Geometry: final body of the model. Coordinates: model frame, mm. A direction names the side the tool comes from. Give positions to 0.01 mm unless a question says otherwise; leave off trailing zeros. Write each loop counter-clockwise with the first axis right and the second up, starting at its lowest first coordinate (ties: lowest second). Pieces come first, ordered by that corner, then holes.
```python
from build123d import *

# Parameters (mm, degrees)
SKETCH1_W                 = 20
SKETCH1_H                 = 10
BOSS_EXTRUDE1_DEPTH       = 90
M4X0_7_TAPPED_HOLE1_D     = 3.3
M4X0_7_TAPPED_HOLE1_DEPTH = 15
M4X0_7_TAPPED_HOLE1_TIP   = 0.991420021
M4X0_7_TAPPED_HOLE2_D     = 3.3
M4X0_7_TAPPED_HOLE2_DEPTH = 15
M4X0_7_TAPPED_HOLE2_TIP   = 0.991420021


with BuildPart() as part:
    # Sketch1 → Boss-Extrude1 (new body)
    with BuildSketch(Plane(origin=(0, 0, 0), x_dir=(1, 0, 0), z_dir=(0, 1, 0))):
        Rectangle(SKETCH1_W, SKETCH1_H)
    extrude(amount=BOSS_EXTRUDE1_DEPTH)

    # M4x0.7 Tapped Hole1
    with Locations(Plane(origin=(0, 0, 0), x_dir=(-1, 0, 0), z_dir=(0, -1, 0))):
        with Locations((-5, 0), (5, 0)):
            Hole(M4X0_7_TAPPED_HOLE1_D / 2, depth=M4X0_7_TAPPED_HOLE1_DEPTH)
            with Locations((0, 0, -(M4X0_7_TAPPED_HOLE1_DEPTH + M4X0_7_TAPPED_HOLE1_TIP / 2))):  # 118° drill point
                Cone(0, M4X0_7_TAPPED_HOLE1_D / 2, M4X0_7_TAPPED_HOLE1_TIP, mode=Mode.SUBTRACT)

    # M4x0.7 Tapped Hole2
    with Locations(Plane(origin=(0, 90, 0), x_dir=(1, 0, 0), z_dir=(0, 1, 0))):
        with Locations((-5, 0), (5, 0)):
            Hole(M4X0_7_TAPPED_HOLE2_D / 2, depth=M4X0_7_TAPPED_HOLE2_DEPTH)
            with Locations((0, 0, -(M4X0_7_TAPPED_HOLE2_DEPTH + M4X0_7_TAPPED_HOLE2_TIP / 2))):  # 118° drill point
                Cone(0, M4X0_7_TAPPED_HOLE2_D / 2, M4X0_7_TAPPED_HOLE2_TIP, mode=Mode.SUBTRACT)


solid = part.part
```
Item 1: Line query: L1, parallel to Z at x = 5, y = 79.5; L2, parallel to Z at x = 6, y = 5; L3, parallel to Y at x = -5, z = -1. Output: solid intervals per line, ascending.
Found:
L1: z = -5 to -1.65, 1.65 to 5
L2: z = -5 to -1.31, 1.31 to 5
L3: y = 15.39 to 74.61
Item 2: Section A-A, the plane y = 11. Return the cut outline in (x, z), plus the area to 3 significant figures.
Found:
outline: (-10, -5) - (10, -5) - (10, 5) - (-10, 5) - close; hole circle Ø3.3 at (-5, 0); hole circle Ø3.3 at (5, 0)
area: 183 mm2
Item 3: Pull-direction query (Z, two-part tool) for faces 4 (the face through (0, 44, -5)), 5 (the face through (-5.286, 74.181, -0.013)), 6 (the face through (0, 90, 0)); classes: +Z half, -Z half, draft (parallel to the pull), parting line (faces both ways), or undercut.
Found:
face 4: -Z half
face 5: undercut
face 6: draft
Item 4: Reachability of faces 1 (the face through (-6.65, 7.6, -0.07)), 2 (the face through (-10, 44, 0)), 3 (the face through (6.65, 82.4, -0.07)) from +Z, -Z, +X, -X, +Y, -Y: full face, straight path, thin tool, end or side. Return the list, or none.
Found:
face 1: -Y
face 2: +Z, -Z, -X, +Y, -Y
face 3: +Y
Item 5: Pin query (flat end, axial travel): pin 1 Ø3 at (x, z) = (-5, 0) entering from +Y; pin 2 Ø2 at (x, z) = (-5, 0) entering from +Y. Return the tip coordinate at first contact, or that it passes through.
Found:
pin 1: stops at y = 74.91
pin 2: stops at y = 74.61
